Could you check a few things on this model? Use its own coordinates, in mm. Face numbers are marked on the shaded views. A direction names the side the tool comes from. Coordinates: 2 decimals unless noted, no trailing zeros. Loops run counter-clockwise (first coordinate to the right, second up) from the corner with the lowest first, then second, coordinate; pieces in that order, holes last. Notation, with made-up numbers: M -15,-26 L 23,-26 A21 ccw 23,-8 Z; hole C 47,-16 d11. An arc over 180 degrees is marked long. Write each question's results on one line, items separated by ' | '.
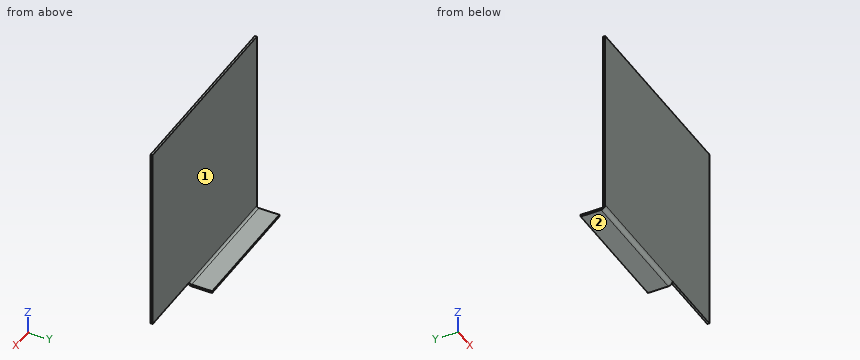
```python
from build123d import *

# Parameters (mm, degrees)
BASE_FLANGE1_DEPTH = 3.175
EDGE_FLANGE1_DEPTH = 195.521520056


# Sheet-metal steps are written as plain solids
with BuildPart() as part:
    # Sketch1 → Base-Flange1 (new body)
    with BuildSketch(Plane(origin=(0, 0, 0), x_dir=(1, 0, 0), z_dir=(0, 1, 0))):
        Polygon((0, 290.83), (-101.6, 290.83), (-101.6, 0), (0, 0), (201.20864, 0), (201.20864, 290.83), align=None)
    extrude(amount=-BASE_FLANGE1_DEPTH)

    # Edge-Flange1 section (across the edge) → Edge-Flange1 (add)
    with BuildSketch(Plane(origin=(93.921520056, 0, -294.005), x_dir=(0, 0, 1), z_dir=(-1, 0, 0))):
        with BuildLine():
            Line((-3.175, 3.175), (-3.175, 34.925))
            Line((-3.175, 34.925), (0, 34.925))
            Line((0, 34.925), (0, 3.175))
            ThreePointArc((0, 3.175), (0.92993597, 0.92993597), (3.175, 0))
            Line((3.175, 0), (3.175, -3.175))
            ThreePointArc((3.175, -3.175), (-1.315128061, -1.315128061), (-3.175, 3.175))
        make_face()
    extrude(amount=EDGE_FLANGE1_DEPTH)


solid = part.part
```
(1) Imagine slicing it at B-B, the plane z = -42.5. List the corners of the cut face in (x, y) for me (3 decimals).
Reported:
outline: M -101.6,-3.175 L 201.209,-3.175 L 201.209,0 L -101.6,0 Z
(2) Which directions (+Z, -Z, +X, -X, +Y, -Y) give clear straight access to the entire face, cutting with the end or side of a thin tool? Please do the marked faces 1 and 2.
Reported:
face 1: +Z, +X, -X, +Y | face 2: -Z, +X, -X, +Y, -Y
(3) Please list where these lines run through material, in increasing order: probe 1 along Z at (x, y) = (25, 31) (3 decimals); probe 2 along Y at (x, z) = (135, -198) (3 decimals); probe 3 along Z at (x, y) = (148.5, -1). Write a range as from..to.
Reported:
probe 1: z = -297.18..-294.005 | probe 2: y = -3.175..0 | probe 3: z = -290.83..0
(4) Imagine slicing it at C-C, the plane y = 11.5. List the corners of the cut face in (x, z) for me (3 decimals).
Reported:
outline: M -101.6,-297.18 L 93.922,-297.18 L 93.922,-294.005 L -101.6,-294.005 Z
(5) Imagine slicing it at A-A, the plane x = -69. List the corners of the cut face in (y, z) for me (3 decimals).
Reported:
outline: M -3.175,-290.83 A6.35 ccw 3.175,-297.18 L 34.925,-297.18 L 34.925,-294.005 L 3.175,-294.005 A3.175 cw 0,-290.83 L 0,0 L -3.175,0 Z
(6) Will these pins go through, and if not, where does the flat tip stop? P1, Ø12, axis at x = -43, z = -111, coming from the +Y side; P2, Ø1.5, axis at x = 92.5, y = 14.5, coming from the +Z side (3 decimals); P3, Ø1.6, axis at x = 173.5, y = -1.5, coming from the -Z side.
Reported:
P1: stops at y = 0 | P2: stops at z = -294.005 | P3: stops at z = -290.83
